Could you check a few things on this drawing? It's one solid part, dimensions in mm from its lowest x, y, z. A direction names the side the tool comes from. Round coordinates to 2 decimals unless told otherwise and drop trailing zeros. Write each loop counter-clockwise with the first axis right and the second up, starting at its lowest first coordinate (ties: lowest second). Pieces come first, ordered by that corner, then holes. Notation, with made-up numbers: (60.5, 63.25) - (86.5, 63.25) arc R21 cw to (86.5, 78.25) - close; hole circle Ø2 at (-7.75, 80.5). An arc over 180 degrees is marked (long way). One line per question, with ' | ' between items. Start each with the question number.
(1) Will these pins go through, and if not, where does the flat tip stop? pin 1 (2 mm diameter, centred on x = 9.5, z = 7.5, fed in from -Y); pin 2 (4 mm diameter, centred on x = 3, z = 8.5, fed in from +Y); pin 3 (6 mm diameter, centred on x = 5, z = 3.5, fed in from -Y).
(2) For the marked faces 4, 5, 6 and 7, which set-ups out of +Z, -Z, +X, -X, +Y, -Y let a thin tool reach every point of the face, with its end or its side?
(3) Thinking about a two-plate mould opening in Z: for the marked faces 1, 2 and 3, which applies, pulls with the +Z half, pulls with the -Z half, needs draft (parallel to the pull), parting line crosses it, or undercut?
(4) Imagine slicing it at D-D (x = 10). Write out the boundary of the cut face in (y, z), plus the area to 3 significant figures.
(5) If I drill on L1, parallel to Y at x = 10, z = 9.3; L2, parallel to Z at x = 6.25, y = 7.25; L3, parallel to X at y = 5.5, z = 0.75, over which ranges is the centre line in solid material (lowest first)?
(6) Imagine slicing it at C-C (x = 6.5). Write out the boundary of the cut face in (y, z).
(7) Imagine slicing it at B-B (z = 5). Write out the boundary of the cut face in (x, y), plus the area to 3 significant figures.
(8) Imagine slicing it at A-A (y = 5.5). Write out the boundary of the cut face in (x, z).
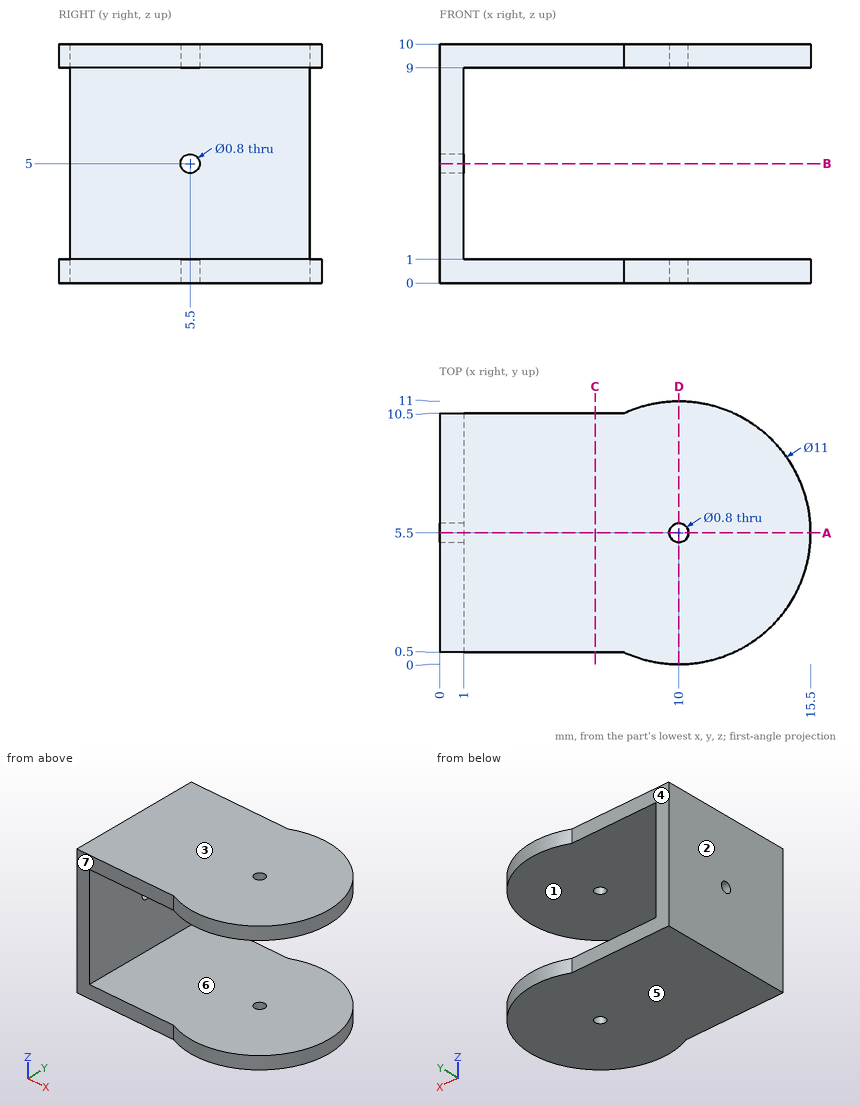
Check sheet entries:
1) pin 1: through | pin 2: y = 10.5 | pin 3: y = 0.5
2) face 4: +Z, -Z, -X, +Y | face 5: -Z, +X, -X, +Y, -Y | face 6: +X, +Y, -Y | face 7: +Z, -Z, -X, -Y
3) face 1: undercut | face 2: needs draft | face 3: pulls with the +Z half
4) outline: (0, 0) - (5.1, 0) - (5.1, 1) - (0, 1) - close; (0, 9) - (5.1, 9) - (5.1, 10) - (0, 10) - close; (5.9, 0) - (11, 0) - (11, 1) - (5.9, 1) - close; (5.9, 9) - (11, 9) - (11, 10) - (5.9, 10) - close | area: 20.4 mm^2
5) L1: 0 to 5.1, 5.9 to 11 | L2: 0 to 1, 9 to 10 | L3: 0 to 9.6, 10.4 to 15.5
6) outline: (0.5, 0) - (10.5, 0) - (10.5, 1) - (0.5, 1) - close; (0.5, 9) - (10.5, 9) - (10.5, 10) - (0.5, 10) - close
7) outline: (0, 0.5) - (1, 0.5) - (1, 5.1) - (0, 5.1) - close; (0, 5.9) - (1, 5.9) - (1, 10.5) - (0, 10.5) - close | area: 9.20 mm^2
8) outline: (0, 0) - (9.6, 0) - (9.6, 1) - (1, 1) - (1, 4.6) - (0, 4.6) - close; (0, 5.4) - (1, 5.4) - (1, 9) - (9.6, 9) - (9.6, 10) - (0, 10) - close; (10.4, 0) - (15.5, 0) - (15.5, 1) - (10.4, 1) - close; (10.4, 9) - (15.5, 9) - (15.5, 10) - (10.4, 10) - close
